Design review of the part built by this model. Coordinates are the model's own, in mm. A direction names the side the tool comes from. Round coordinates to 2 decimals unless told otherwise and drop trailing zeros. Write each loop counter-clockwise with the first axis right and the second up, starting at its lowest first coordinate (ties: lowest second). Pieces come first, ordered by that corner, then holes. Notation, with made-up numbers: M 17.25,35 L 76.25,35 A24 ccw 76.25,63 Z; hole C -12.75,17.5 d1. An arc over 180 degrees is marked long. Use CSV: the item, a comma, the result in double quotes.
from build123d import *
from build123d.topology import SkipClean

# Parameters (mm, degrees)
BOSS_EXTRUDE4_DEPTH            = 4
BOSS_EXTRUDE4_2_DEPTH          = 4
BOSS_EXTRUDE7_START            = 4
SKETCH13_W                     = 77
SKETCH13_H                     = 2
BOSS_EXTRUDE7_DEPTH            = 2
CUT_EXTRUDE3_REACH             = 87.589
SKETCH11_W                     = 2
SKETCH11_H                     = 2.2
CUT_EXTRUDE3_DIRECTION_2_REACH = 87.589
BOSS_EXTRUDE6_DEPTH            = 2
M3_CLEARANCE_HOLE1_D           = 3.6
SKETCH16_R                     = 3
CUT_EXTRUDE4_DEPTH             = 2
CHAMFER2_SIZE                  = 2
CHAMFER3_SIZE                  = 0.5


with BuildPart() as part:
    # Sketch9 → Boss-Extrude4 (new body)
    with BuildSketch(Plane.XY):
        with BuildLine():
            Line((-60.736133913, -37.540305051), (-42.5, -27.622167018))
            Line((-42.5, -27.622167018), (-42.5, 27.622167018))
            Line((-42.5, 27.622167018), (-60.736133913, 37.540305051))
            ThreePointArc((-60.736133913, 37.540305051), (-70.020874221, 44.866685358), (-58.825010341, 41.054221199))
            Line((-58.825010341, 41.054221199), (-38.5, 30))
            Line((-38.5, 30), (-38.5, -30))
            Line((-38.5, -30), (-58.825010341, -41.054221199))
            ThreePointArc((-58.825010341, -41.054221199), (-70.020874221, -44.866685358), (-60.736133913, -37.540305051))
        make_face()
    extrude(amount=BOSS_EXTRUDE4_DEPTH)



with BuildPart() as body_2:
    # Sketch9 → Boss-Extrude4 2 (new body)
    with BuildSketch(Plane.XY):
        with BuildLine():
            Line((38.5, -30), (58.825010341, -41.054221199))
            ThreePointArc((58.825010341, -41.054221199), (70.020874221, -44.866685358), (60.736133913, -37.540305051))
            Line((60.736133913, -37.540305051), (42.5, -27.622167018))
            Line((42.5, -27.622167018), (42.5, 27.622167018))
            Line((42.5, 27.622167018), (60.736133913, 37.540305051))
            ThreePointArc((60.736133913, 37.540305051), (70.020874221, 44.866685358), (58.825010341, 41.054221199))
            Line((58.825010341, 41.054221199), (38.5, 30))
            Line((38.5, 30), (38.5, -30))
        make_face()
    extrude(amount=BOSS_EXTRUDE4_2_DEPTH)


with BuildPart() as part_1:
    add(part.part)

    add(body_2.part)  # Boss-Extrude7 merges body 2
    # Sketch13 → Boss-Extrude7 (add)
    with BuildSketch(Plane.XY.offset(BOSS_EXTRUDE7_START)):
        with Locations((0, -29)):
            Rectangle(SKETCH13_W, SKETCH13_H)
    extrude(amount=-BOSS_EXTRUDE7_DEPTH)

    # Cut-Extrude3: up to this face of the body (flat: up to its plane)
    cut_extrude3_end = Plane(part_1.part.faces().sort_by_distance((0, -28, 3))[0])
    # Sketch11 → Cut-Extrude3 (cut, up to the picked face)
    with BuildSketch(Plane(origin=(0, 0, 0), x_dir=(1, 0, 0), z_dir=(0, 1, 0)), mode=Mode.PRIVATE) as cut_extrude3_sk1:
        with Locations((-39.5, -2.9)):
            Rectangle(SKETCH11_W, SKETCH11_H)
    cut_extrude3_tool1 = split(extrude(cut_extrude3_sk1.sketch, amount=-CUT_EXTRUDE3_REACH, mode=Mode.PRIVATE), bisect_by=cut_extrude3_end, keep=Keep.BOTH, mode=Mode.PRIVATE)
    # Sketch11 → Cut-Extrude3 (cut, up to the picked face)
    with BuildSketch(Plane(origin=(0, 0, 0), x_dir=(1, 0, 0), z_dir=(0, 1, 0)), mode=Mode.PRIVATE) as cut_extrude3_sk2:
        with Locations((39.5, -2.9)):
            Rectangle(SKETCH11_W, SKETCH11_H)
    cut_extrude3_tool2 = split(extrude(cut_extrude3_sk2.sketch, amount=-CUT_EXTRUDE3_REACH, mode=Mode.PRIVATE), bisect_by=cut_extrude3_end, keep=Keep.BOTH, mode=Mode.PRIVATE)
    add(cut_extrude3_tool1.solids().sort_by(Axis((-39.5, 0, 2.9), (0, -1, 0)))[0], mode=Mode.SUBTRACT)
    add(cut_extrude3_tool2.solids().sort_by(Axis((39.5, 0, 2.9), (0, -1, 0)))[0], mode=Mode.SUBTRACT)

    # Sketch11 → Cut-Extrude3 direction 2 (cut, up to next)
    with BuildSketch(Plane(origin=(0, 0, 0), x_dir=(1, 0, 0), z_dir=(0, 1, 0)), mode=Mode.PRIVATE) as cut_extrude3_direction_2_sk1:
        with Locations((-39.5, -2.9)):
            Rectangle(SKETCH11_W, SKETCH11_H)
    cut_extrude3_direction_2_tool1 = extrude(cut_extrude3_direction_2_sk1.sketch, amount=CUT_EXTRUDE3_DIRECTION_2_REACH, mode=Mode.PRIVATE) & part_1.part
    # Sketch11 → Cut-Extrude3 direction 2 (cut, up to next)
    with BuildSketch(Plane(origin=(0, 0, 0), x_dir=(1, 0, 0), z_dir=(0, 1, 0)), mode=Mode.PRIVATE) as cut_extrude3_direction_2_sk2:
        with Locations((39.5, -2.9)):
            Rectangle(SKETCH11_W, SKETCH11_H)
    cut_extrude3_direction_2_tool2 = extrude(cut_extrude3_direction_2_sk2.sketch, amount=CUT_EXTRUDE3_DIRECTION_2_REACH, mode=Mode.PRIVATE) & part_1.part
    add(cut_extrude3_direction_2_tool1.solids().sort_by_distance((-39.5, 0, 2.9))[0], mode=Mode.SUBTRACT)
    add(cut_extrude3_direction_2_tool2.solids().sort_by_distance((39.5, 0, 2.9))[0], mode=Mode.SUBTRACT)

    # Sketch12 → Boss-Extrude6 (add)
    with SkipClean():  # the faces are left unmerged after this step: merging them gives an invalid solid
        with BuildSketch(Plane.XY.offset(4)):
            with BuildLine():
                Line((-67.616685358, 36.729125779), (-46.5, 25.244334036))
                Line((-46.5, 25.244334036), (-46.5, -25.244334036))
                Line((-46.5, -25.244334036), (-67.616685358, -36.729125779))
                ThreePointArc((-67.616685358, -36.729125779), (-70.020874221, -44.866685358), (-61.883314642, -47.270874221))
                Line((-61.883314642, -47.270874221), (-41.159951957, -36))
                Line((-41.159951957, -36), (41.159951957, -36))
                Line((41.159951957, -36), (61.883314642, -47.270874221))
                ThreePointArc((61.883314642, -47.270874221), (70.020874221, -44.866685358), (67.616685358, -36.729125779))
                Line((67.616685358, -36.729125779), (46.5, -25.244334036))
                Line((46.5, -25.244334036), (46.5, 25.244334036))
                Line((46.5, 25.244334036), (67.616685358, 36.729125779))
                ThreePointArc((67.616685358, 36.729125779), (70.020874221, 44.866685358), (61.883314642, 47.270874221))
                Line((61.883314642, 47.270874221), (41.159951957, 36))
                Line((41.159951957, 36), (-41.159951957, 36))
                Line((-41.159951957, 36), (-61.883314642, 47.270874221))
                ThreePointArc((-61.883314642, 47.270874221), (-70.020874221, 44.866685358), (-67.616685358, 36.729125779))
            make_face()
        extrude(amount=BOSS_EXTRUDE6_DEPTH)

    # M3 Clearance Hole1 (through all)
    with Locations(Plane(origin=(0, 0, 0), x_dir=(-1, 0, 0), z_dir=(0, 0, -1))):
        with Locations((64.75, 42), (64.75, -42), (-64.75, -42), (-64.75, 42)):
            Hole(M3_CLEARANCE_HOLE1_D / 2)

    # Sketch16 → Cut-Extrude4 (cut)
    with SkipClean():  # the faces are left unmerged after this step: merging them gives an invalid solid
        with BuildSketch(Plane.XY.offset(6)):
            with Locations((-64.75, 42)):
                Circle(SKETCH16_R)
            with Locations((-64.75, -42)):
                Circle(SKETCH16_R)
            with Locations((64.75, -42)):
                Circle(SKETCH16_R)
            with Locations((64.75, 42)):
                Circle(SKETCH16_R)
        extrude(amount=-CUT_EXTRUDE4_DEPTH, mode=Mode.SUBTRACT)

    # Chamfer2
    chamfer2_edges = [part_1.edges().sort_by_distance(p)[0] for p in [
        (-49.662505171, 36.070983444, 4),
        (49.662505171, 36.070983444, 4),
        (51.618066957, 32.581236035, 4),
        (42.5, 0, 4),
        (51.618066957, -32.581236035, 4),
        (48.662505171, -35.527110599, 4),
        (-48.662505171, -35.527110599, 4),
        (-51.618066957, -32.581236035, 4),
        (-51.618066957, 32.581236035, 4),
        (-42.5, 0, 4),
        (0, -30, 4),
    ]]
    chamfer(chamfer2_edges, length=CHAMFER2_SIZE - 0.0001)  # a hair under: the kernel refuses the full size

    # Chamfer3
    chamfer3_edges = [part_1.edges().sort_by_distance(p)[0] for p in [
        (-38.5, 0, 0),
        (38.5, 0, 0),
    ]]
    chamfer(chamfer3_edges, length=CHAMFER3_SIZE)


solid = part_1.part
1) Add section A-A on x = -49. Write out the cut boundary in (y, z), then the cut area to 3 significant figures.
Answers:
outline,"M -40.26,4 L -37.99,4 L -35.71,2 L -35.71,0 L -31.16,0 L -31.16,2 L -28.88,4 L -26.6,4 L -26.6,6 L -40.26,6 Z; M 26.6,4 L 28.88,4 L 31.16,2 L 31.16,0 L 35.71,0 L 35.71,2 L 37.99,4 L 40.26,4 L 40.26,6 L 26.6,6 Z"
area,"100 mm²"
2) Wall thickness on line 1 along Y through (x, z) = (-64.75, 1.8); line 2 along Z through (x, y) = (39, -6.5); line 3 along X through (y, z) = (-36.5, 1.5): over which ranges is each line inside the solid? List them lowest first. Write a range as [from, to].
Answers:
line 1,"[-48, -43.8], [-40.2, -36], [36, 40.2], [43.8, 48]"
line 2,"[0, 1.8], [4, 6]"
line 3,"[-67.15, -62.35], [-58.82, -50.45], [50.45, 58.82], [62.35, 67.15]"
3) Machinability: for faces 5 (the face through (-57.21, 31.07, 4.99)), 6 (the face through (-51.38, 41.56, 4.99)), 7 (the face through (-1, 1, 6)), 8 (the face through (62.54, -39.97, 5.01)), which of the approach directions +Z, -Z, +X, -X, +Y, -Y give a long, thin tool a straight path to every point of the face, cutting with its end or side? Answer none if there is none.
Answers:
face 5,"+Z, -Z, -X"
face 6,"+Z, -Z, +Y"
face 7,"+Z, +X, -X, +Y, -Y"
face 8,"+Z"
4) Add section C-C on y = -14.5. Write out the cut boundary in (x, z), then the cut area to 3 significant figures.
Answers:
outline,"M -46.5,4 L -44.5,4 L -42.5,2 L -42.5,0 L -39,0 L -38.5,0.5 L -38.5,1.8 L -40.5,1.8 L -40.5,4 L 40.5,4 L 40.5,1.8 L 38.5,1.8 L 38.5,0.5 L 39,0 L 42.5,0 L 42.5,2 L 44.5,4 L 46.5,4 L 46.5,6 L -46.5,6 Z"
area,"213 mm²"
5) For pin 1 Ø0.6 at (x, z) = (8, 5) entering from +Y; pin 2 Ø0.5 at (y, z) = (-12, 1) entering from +X; pin 3 Ø5.5 at (x, y) = (-64.75, 42) entering from +Z; pin 4 Ø10 at (x, y) = (-45.5, 17.5) entering from -Z, all flat-tipped, find the tip position at first contact; note any pin that passes through.
Answers:
pin 1,"y = 36"
pin 2,"x = 42.5"
pin 3,"z = 4"
pin 4,"z = 0"
6) The part is to be moulded in two halves that separate along Y. For faces 1 (the face through (-46, 0, 4)), 2 (the face through (-51.667, -41.714, 4.986)), 3 (the face through (42, 4, 0)), 4 (the face through (-66.96, 44.03, 5.01)), say which applies: released by +Y, released by -Y, zero draft, split by the parting line, or undercut.
Answers:
face 1,"undercut"
face 2,"released by -Y"
face 3,"zero draft"
face 4,"undercut"
7) Add section B-B on z = 5. Write out the cut boundary in (x, y), then the cut area to 3 significant figures.
Answers:
outline,"M -67.62,-36.73 A6 ccw -61.88,-47.27 L -41.16,-36 L 41.16,-36 L 61.88,-47.27 A6 ccw 67.62,-36.73 L 46.5,-25.24 L 46.5,25.24 L 67.62,36.73 A6 ccw 61.88,47.27 L 41.16,36 L -41.16,36 L -61.88,47.27 A6 ccw -67.62,36.73 L -46.5,25.24 L -46.5,-25.24 Z; hole C -64.75,-42 d6; hole C -64.75,42 d6; hole C 64.75,-42 d6; hole C 64.75,42 d6"
area,"7,840 mm²"
